Check sheet for the modelled part. Datum: model origin and axes. Units: mm. A direction names the side the tool comes from. Round coordinates to 2 decimals unless told otherwise and drop trailing zeros. Write each loop counter-clockwise with the first axis right and the second up, starting at its lowest first coordinate (ties: lowest second). Pieces come first, ordered by that corner, then holes. Notation, with made-up numbers: (-20.75, 57.5) -> (14.25, 57.5) arc R24 ccw to (14.25, 77.5) -> close; hole circle Ø4 at (65.5, -14.5). An arc over 180 degrees is marked (long way). Use one line per item in the form item = value. Start each with the question number.
Autodesk Inventor part; units mm, degrees
ref_plane "Work Plane1" through (14, 0, 0) normal (0, 1, 0) x (1, 0, 0)
ref_plane "Work Plane2" through (14, 0, 0) normal (0, 0, 1) x (1, 0, 0)
ref_plane "YZ Plane" through (0, 0, 0) normal (1, 0, 0) x (0, 1, 0)
sketch "Szkic1" plane through (0, 0, 0) normal (0, 0, 1) x (1, 0, 0)
  line L0 (-13, 0) -> (-13, 7)
  line L1 (-13, 7) -> (-12, 17.5)
  line L2 (-12, 17.5) -> (0, 17.5)
  line L3 (0, 17.5) -> (0, 8)
  line L4 (0, 8) -> (28, 8)
  line L5 (28, 8) -> (28, 0)
  line L6 (28, 0) -> (-13, 0)
  line L7 (-21.2, 0) -> (36.2, 0)
  line L8 (0, -3.5) -> (0, 21)
  dimension "d0" = 16
  dimension "d1" = 35
  dimension "d2" = 28
  dimension "d3" = 12
  dimension "d4" = 14
  dimension "d15" = 13
revolve "Bryła" add sketch "Szkic1" angle 360 about axis through (28, 0, 0) along (-1, 0, 0)
thread "Gwint1"
chamfer "Faza1" distance 1.2269 distance2 1.2269 1 edges at (28, -8, 0) measured on face at (28, 2.3612, -1.2393)
sketch "Szkic2" plane through (0, 0, 0) normal (0, 1, 0) x (-1, 0, 0)
  line L0 (69.6, 0) -> (-11.6, 0)
  line L1 (0, -9.8) -> (0, 9.8)
  circle A0 centre (51, 0) radius 7
  line L2 (51, 7) -> (0, 7) construction
  line L3 (51, -7) -> (0, -7) construction
  line L4 (32, 7) -> (32, -7)
  dimension "d12" = 14
  dimension "d13" = 58
  dimension "d14" = 32
revolve "Oczko" add sketch "Szkic2" angle 360 about axis through (-32, 0, 7) along (0, 0, -1)
ref_plane "Work Plane1" through (14, 0, 0) normal (0, 1, 0) x (1, 0, 0)
ref_plane "Work Plane2" through (14, 0, 0) normal (0, 0, 1) x (1, 0, 0)
equation "\"d0\" = GD"
equation "\"d1\" = LADI"
equation "\"d2\" = NLG"
equation "\"d3\" = KOH1"
equation "\"d4\" = SDR1"
equation "\"d15\" = -SD1 + KOH - 1.5 * SDR1"
equation "\"d5\" = GEL"
equation "\"d7\" = -0.5 * GD1 + 0.5 * GD"
equation "\"d8\" = GUL"
equation "\"d12\" = SDR1"
equation "\"d13\" = KOH"
equation "\"d14\" = DSH"
equation "\"NLG\" = 28"
equation "\"GD\" = NND"
equation "\"LADI\" = 35"
equation "\"KOH1\" = 12"
equation "\"KOH\" = 58"
equation "\"DSH\" = 32"
equation "\"GEL\" = 24"
equation "\"GD1\" = THREADDIA - 1.2269 * PTC"
equation "\"GUL\" = 0.61345 * PTC"
equation "\"SDR1\" = 14"
equation "\"SD1\" = 24"
equation "\"PTC\" = 2"
equation "\"GAL\" = 0.61345 * PTC"
equation "\"THREADDIA\" = 16"
equation "\"SDR2\" = SDR1"
equation "\"TOA\" = 30deg"
equation "\"RR\" = 12"
equation "\"RR2\" = 1"
equation "\"NND\" = 16"
equation "\"GAL2\" = 4"
equation "\"SD2\" = 52"
properties part number "AS 2317 - M16" material "Stal, miękka"
1. Sectioned sample at C-C (x = 15.5). Enter the section's corners in (y, z), and give its area (3 significant figures).
2. Depth check by flat-ended pin: pin 1 (3 mm diameter, centred on y = 20.5, z = 6, fed in from +X); pin 2 (6 mm diameter, centred on x = 7, z = -3, fed in from -Y); pin 3 (2 mm diameter, centred on x = -20, y = 4, fed in from +Z). Enter the tip coordinate at first touch or a pass-through.
3. Scan lines: probe 1 along Y at (x, z) = (-22, 1); probe 2 along X at (y, z) = (4, 2); probe 3 along Y at (x, z) = (-10, 0). Record each from-to range of solid material in increasing order.
4. Sectioned sample at A-A (y = 0). Enter the section's corners in (x, z), and give its area (3 significant figures).
5. Tool access check on faces 1 (the face through (28, 0, 0)), 2 (the face through (13.57, -1.73, -7.81)), 3 (the face through (-12.937, -1.66, -7.475)). Record the directions out of +Z, -Z, +X, -X, +Y, -Y that give a thin tool (end or side, any length) a straight path to the whole face; none if there is none.
6. Sectioned sample at B-B (x = -5). Enter the section's corners in (y, z).
Returned:
q1.outline = circle Ø16 at (0, 0)
q1.area = 201 mm^2
q2.pin_1 = -17.98
q2.pin_2 = -8
q2.pin_3 = 4.51
q3.probe_1 = -23.92 to -6.76, 6.76 to 23.92
q3.probe_2 = -57.4 to -43.62, -20.38 to 28
q3.probe_3 = -17.5 to 17.5
q4.outline = circle Ø14 at (-51, 0); (-13, -7) -> (-12, -17.5) -> (0, -17.5) -> (0, -8) -> (26.77, -8) -> (28, -6.77) -> (28, 6.77) -> (26.77, 8) -> (0, 8) -> (0, 17.5) -> (-12, 17.5) -> (-13, 7) arc R7 ccw to start
q4.area = 1,120 mm^2
q5.face_1 = +Z, -Z, +X, +Y, -Y
q5.face_2 = +X
q5.face_3 = none
q6.outline = circle Ø35 at (0, 0)
